The model under review builds one solid part; all positions refer to its coordinate system, in mm. A direction names the side the tool comes from. Coordinates: 2 decimals unless noted, no trailing zeros. Loops run counter-clockwise (first coordinate to the right, second up) from the corner with the lowest first, then second, coordinate; pieces in that order, holes last. Notation, with made-up numbers: (-23, 87.25) - (19, 87.25) arc R36 cw to (19, 123.25) - close; hole circle Ø4 at (-22, -25.75). An arc over 180 degrees is marked (long way). Use a Markdown table: item, result. Add a question column.
1) To check wall thickness, follow L1, parallel to Y at x = 12.5, z = -0.05; L2, parallel to X at y = -0.85, z = -0.35. State the ranges of each line that lie inside material, in increasing order. Write a range as [from, to].
2) The part is to be moulded in two halves that separate along Y. For faces 3 (the flat face through (-1.41, -0.5, -0.86)), 4 (the cylindrical face through (10.85, -1.5, -0.07)), 5 (the flat face through (22, 0, 0)), say which applies: pulls with the +Y half, pulls with the -Y half, needs draft (parallel to the pull), parting line crosses it, or undercut.
3) Add section A-A, the plane x = 18.5. Give the boundary of the cut face in (y, z), and give its area (3 significant figures).
4) Clearance check with flat-ended pins moving along their axes: pin 1 (1.3 mm diameter, centred on x = -1.5, z = 0, fed in from -Y); pin 2 (0.9 mm diameter, centred on x = -1.5, z = 0, fed in from +Y); pin 3 (1 mm diameter, centred on x = 11.5, y = 1, fed in from -Z). State where each tip first meets the part, or that it passes through.
5) For faces 1 (the flat face through (0, 2, 0)), 2 (the flat face through (-1.408, -0.491, 0.867)), list the 3-axis set-ups (+Z, -Z, +X, -X, +Y, -Y) from which the entire face can be reached by the end or side of a thin tool; tool diameter is ignored.
Autodesk Inventor part; units mm, degrees
ref_plane "YZ Plane" through (0, 0, 0) normal (1, 0, 0) x (0, 1, 0)
ref_plane "XZ Plane" through (0, 0, 0) normal (0, 1, 0) x (-1, 0, 0)
ref_plane "XY Plane" through (0, 0, 0) normal (0, 0, 1) x (1, 0, 0)
sketch "スケッチ1" plane through (0, 0, 0) normal (0, 0, 1) x (1, 0, 0)
  line L0 (0, 0) -> (22, 0)
  line L1 (22, 0) -> (22, 1.5)
  line L2 (22, 1.5) -> (0, 1.5)
  line L3 (0, 1.5) -> (0, 0)
  line L4 (0, 0) -> (0, 2.75)
  line L5 (0, 0) -> (-2, 0)
  line L6 (-2, 0) -> (0, 0)
  line L7 (-2, 0) -> (-2, 1.15)
  arc A0 (0, 2.75) -> (-2, 1.15) centre (-0.0403, 0.7504) ccw
  dimension "d0" = 1.5
  dimension "d1" = 22
  dimension "d3" = 2
  dimension "d4" = 2.75
  dimension "d5" = 1.15
  dimension "d6" = 2
revolve "回転1" add sketch "スケッチ1" angle 360 about axis through (-2, 0, 0) along (1, 0, 0)
thread "ねじ1"
sketch "スケッチ2" plane through (-2, 0, 0) normal (-1, 0, 0) x (0, 0, 1)
  circle A0 centre (0, 0) radius 1.15
  line L0 (-0.575, 0.9959) -> (0.575, 0.9959)
  line L1 (0.575, 0.9959) -> (1.15, 0)
  line L2 (1.15, 0) -> (0.575, -0.9959)
  line L3 (0.575, -0.9959) -> (-0.575, -0.9959)
  line L4 (-0.575, -0.9959) -> (-1.15, 0)
  line L5 (-1.15, 0) -> (-0.575, 0.9959)
  dimension "d10" = 1.15
  dimension "d11" = 1.9919
extrude "押し出し1" cut sketch "スケッチ2" against normal blind 1.4 contours L2 L3 L4 L5 L0 L1
fillet "フィレット1" radius 0.2 6 edges at (-0.6, 0.9959, 0) (-0.6, 0.498, 0.8625) (-0.6, 0.498, -0.8625) (-0.6, -0.498, -0.8625) (-0.6, -0.9959, 0) (-0.6, -0.498, 0.8625)
fillet "フィレット2" radius 0.1 1 edges at (0, -1.5, 0)
fillet "フィレット3" radius 0.1 1 edges at (22, -1.5, 0)
properties part number "ネジボタンM3L22" material "鋼"
From the geometry:
| question | item | result |
|---|---|---|
| 1 | L1 | y = [-1.5, 1.5] |
| 1 | L2 | x = [-0.61, 22] |
| 2 | face 3 | undercut |
| 2 | face 4 | parting line crosses it |
| 2 | face 5 | needs draft |
| 3 | outline | circle Ø3 at (0, 0) |
| 3 | area | 7.07 mm^2 |
| 4 | pin 1 | stops at y = -2.58 |
| 4 | pin 2 | stops at y = 2.48 |
| 4 | pin 3 | stops at z = -1.41 |
| 5 | face 1 | +X |
| 5 | face 2 | -X |
